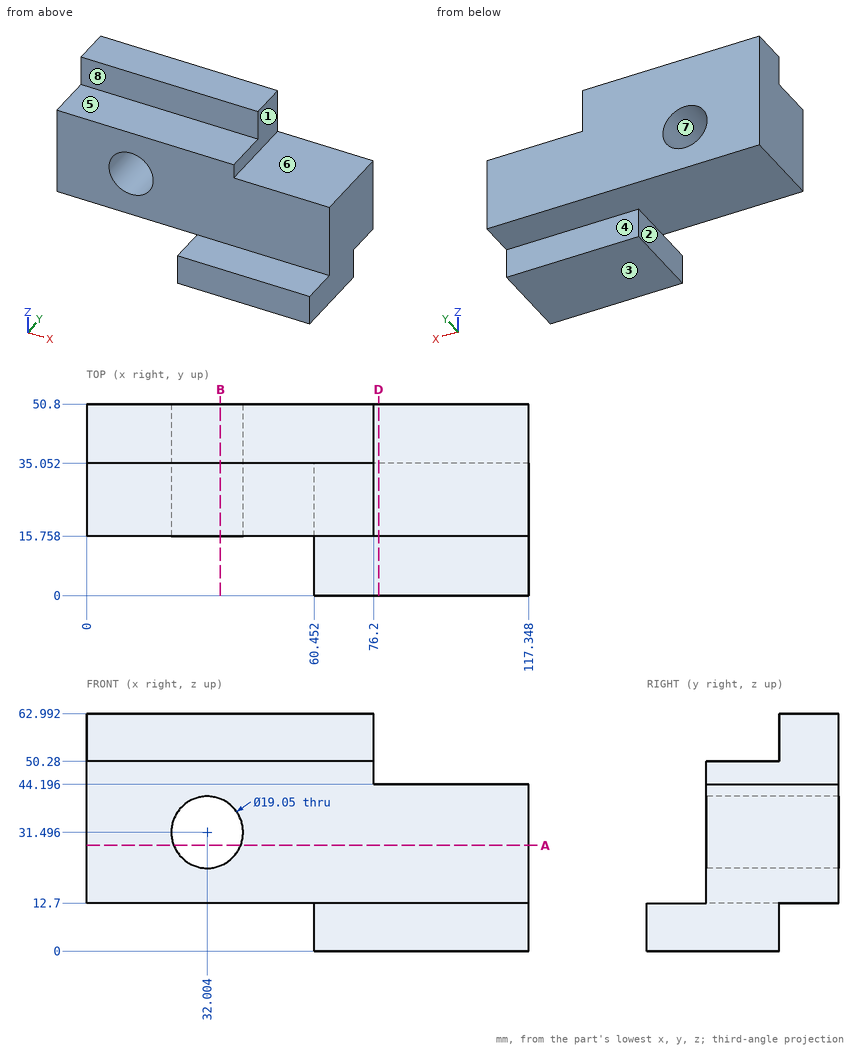
Drawing for the job (mm, zero at the part's lowest x, y, z). A direction names the side the tool comes from. Give positions to 0.01 mm unless a question says otherwise; leave off trailing zeros. Order: outer loops, then holes, each group sorted by start corner. A loop starts at its lowest first (then second) coordinate and runs counter-clockwise, first axis right, second up. Notation, with made-up numbers: (32, 17.5) - (58, 17.5) arc R28 ccw to (58, 39.5) - close; hole circle Ø1 at (-27.5, -34.75). An arc over 180 degrees is marked (long way). Write item = value, one per line. Start each with the question number.
1. Two-plate mould, pull along Z, no slides. Class the marked faces 6, 7 and 8: pulls with the +Z half, pulls with the -Z half, needs draft (parallel to the pull), parting line crosses it, or undercut.
2. Cut at D-D, the plane x = 77.5. List the corners of the cut face in (y, z).
3. Which spindle directions (+Z, -Z, +X, -X, +Y, -Y) get a long thin tool onto all of the face, cutting with end or side? Do the marked faces 1, 2, 3, 4 and 5. Say none if no direction does.
4. Cut at A-A, the plane z = 28. List the corners of the cut face in (x, y) (1 decimal).
5. Probe line 1 along Y through (x, z) = (36, 15.5); line 2 along Z through (x, y) = (97.5, 3.5); line 3 along Z through (x, y) = (71.5, 32). List the from-to ranges inside material, lowest first.
6. Drop flat-ended pins along their axis: P1, Ø4, axis at x = 62, z = 31, coming from the -Y side; P2, Ø4, axis at x = 79.5, z = 8.5, coming from the +Y side; P3, Ø8, axis at x = 55.5, y = 15, coming from the +Z side; P4, Ø11.5, axis at x = 32.004, z = 31.496, coming from the -Y side. Give the stop position or say it passes through.
7. Cut at B-B, the plane x = 35.5. List the corners of the cut face in (y, z) (1 decimal).
Taken from the geometry:
q1.face_6 = pulls with the +Z half
q1.face_7 = undercut
q1.face_8 = needs draft
q2.outline = (0, 0) - (35.05, 0) - (35.05, 12.7) - (50.8, 12.7) - (50.8, 44.2) - (15.76, 44.2) - (15.76, 12.7) - (0, 12.7) - close
q3.face_1 = +Z, +X, +Y, -Y
q3.face_2 = -Z, -X, +Y, -Y
q3.face_3 = -Z, +X, -X, +Y, -Y
q3.face_4 = -Z, +X, -X, +Y
q3.face_5 = +Z, +X, -X, -Y
q4.outline = (0, 15.8) - (23.1, 15.8) - (23.1, 50.8) - (0, 50.8) - close; (40.9, 15.8) - (117.3, 15.8) - (117.3, 50.8) - (40.9, 50.8) - close
q5.line_1 = 15.76 to 50.8
q5.line_2 = 0 to 12.7
q5.line_3 = 0 to 50.28
q6.P1 = 15.76
q6.P2 = 35.05
q6.P3 = 50.28
q6.P4 = through
q7.outline = (15.8, 12.7) - (50.8, 12.7) - (50.8, 22.6) - (15.8, 22.6) - close; (15.8, 40.4) - (50.8, 40.4) - (50.8, 63) - (35.1, 63) - (35.1, 50.3) - (15.8, 50.3) - close
